Here's how the part is built. I have some questions about the finished solid (model axes, mm). Round coordinates to 2 decimals unless told otherwise and drop trailing zeros. Write each loop counter-clockwise with the first axis right and the second up, starting at its lowest first coordinate (ties: lowest second). Pieces come first, ordered by that corner, then holes. Notation, with made-up numbers: (-34, 26) - (-20, 26) arc R25 cw to (-20, 58) - close; hole circle Ø5 at (-0.5, -30.75). An arc over 180 degrees is marked (long way). One line per item, written item: value. Start each with the question number.
Item 1: Imagine slicing it at A-A, the plane z = 10.5. Please give me the cut outline in (x, y), then the cut area to 3 significant figures.
Item 2: Imagine slicing it at B-B, the plane z = 22.25. Please give me the cut outline in (x, y).
Item 3: If I drill on line 1 (Y direction, x = -34, z = 3.75); line 2 (Y direction, x = -42, z = 21.75); line 3 (X direction, y = 2, z = 7.25), over which ranges is the centre line in solid material (lowest first)?
Item 4: For P1, Ø8, axis at x = 17, z = 18, coming from the -Y side; P2, Ø5, axis at x = -17.5, y = -15, coming from the +Z side; P3, Ø5, axis at y = -27, z = 21.5, coming from the -X side, each with a flat end and sliding along its axis, tell me the tip position at first contact or that it passes through.
```python
from build123d import *

# Parameters (mm, degrees)
F1_DEPTH = 25.4
F2_R     = 5


with BuildPart() as f1:
    # F0 (on Top) → F1 (new body)
    with BuildSketch(Plane.XY):
        Polygon((55, 50), (-56, 50), (-56, 18.093373), (18, -44), (55, -44), align=None)
    extrude(amount=F1_DEPTH)

    # F2
    f2_edges = [f1.edges().sort_by_distance(p)[0] for p in [
        (-0.5, 50, 0),
        (-56, 34.046686, 0),
        (-19, -12.953314, 0),
        (36.5, -44, 0),
        (55, 3, 0),
        (-0.5, 50, 25.4),
        (-56, 34.046686, 25.4),
        (-19, -12.953314, 25.4),
        (36.5, -44, 25.4),
        (55, 3, 25.4),
        (-56, 50, 12.7),
        (55, 50, 12.7),
        (-56, 18.093373, 12.7),
        (18, -44, 12.7),
        (55, -44, 12.7),
    ]]
    fillet(f2_edges, radius=F2_R)


solid = f1.part
```
Values follow:
1. outline: (-56, 20.42) arc R5 ccw to (-54.21, 16.59) - (16.61, -42.83) arc R5 ccw to (19.82, -44) - (50, -44) arc R5 ccw to (55, -39) - (55, 45) arc R5 ccw to (50, 50) - (-51, 50) arc R5 ccw to (-56, 45) - close
1. area: 8,120 mm^2
2. outline: (-55.65, 20.42) arc R4.65 ccw to (-53.99, 16.87) - (16.83, -42.56) arc R4.65 ccw to (19.82, -43.65) - (50, -43.65) arc R4.65 ccw to (54.65, -39) - (54.65, 45) arc R4.65 ccw to (50, 49.65) - (-51, 49.65) arc R4.65 ccw to (-55.65, 45) - close
3. line 1: y = -0.16 to 49.84
3. line 2: y = 6.59 to 49.81
3. line 3: x = -36.82 to 55
4. P1: stops at y = -44
4. P2: stops at z = 24.32
4. P3: stops at x = -5.12
